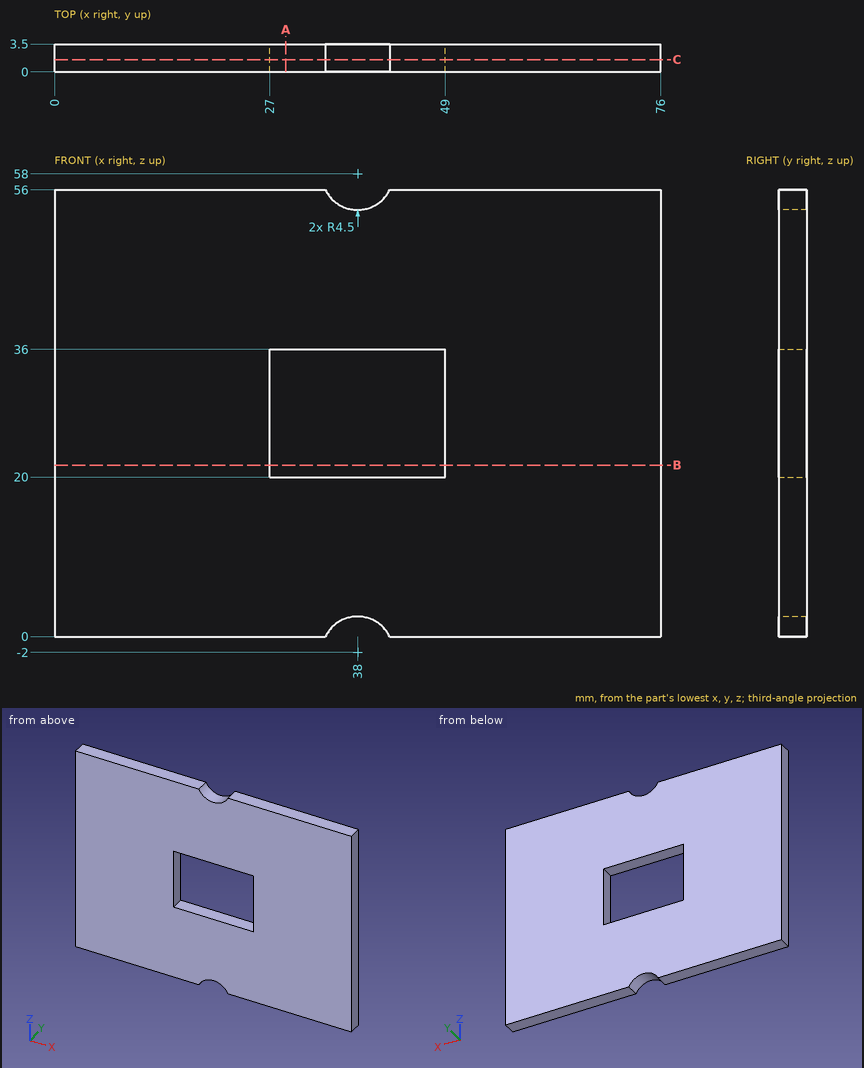
Here's the drawing with two shaded views (mm, measured from the low corner). I have some questions. Round coordinates to 2 decimals unless told otherwise and drop trailing zeros. Loops run counter-clockwise (first coordinate to the right, second up) from the corner with the lowest first, then second, coordinate; pieces in that order, holes last.
Item 1: Suppose I cut it at A-A, the plane x = 29. Write out the boundary of the cut face in (y, z).
Item 2: Suppose I cut it at C-C, the plane y = 1.55. Write out the boundary of the cut face in (x, z), then the cut area to 3 significant figures.
Item 3: Will these pins go through, and if not, where does the flat tip stop? pin 1 Ø1 at (x, y) = (38.5, 2.5) entering from +Z; pin 2 Ø1.8 at (x, y) = (39.5, 2.5) entering from -Z.
Item 4: Please list where these lines run through material, in increasing order: L1, parallel to X at y = 3.15, z = 35; L2, parallel to Z at x = 38, y = 1.15; L3, parallel to Z at x = 32, y = 1.5.
Item 5: Suppose I cut it at B-B, the plane z = 21.5. Write out the boundary of the cut face in (x, y), then the cut area to 3 significant figures.
Reported:
1. outline: (0, 0) - (3.5, 0) - (3.5, 20) - (0, 20) - close; (0, 36) - (3.5, 36) - (3.5, 56) - (0, 56) - close
2. outline: (0, 0) - (33.97, 0) arc R4.5 cw to (42.03, 0) - (76, 0) - (76, 56) - (42.03, 56) arc R4.5 cw to (33.97, 56) - (0, 56) - close; hole (27, 20) - (49, 20) - (49, 36) - (27, 36) - close
2. area: 3,880 mm2
3. pin 1: stops at z = 53.61
3. pin 2: stops at z = 1.81
4. L1: x = 0 to 27, 49 to 76
4. L2: z = 2.5 to 20, 36 to 53.5
4. L3: z = 0 to 20, 36 to 56
5. outline: (0, 0) - (27, 0) - (27, 3.5) - (0, 3.5) - close; (49, 0) - (76, 0) - (76, 3.5) - (49, 3.5) - close
5. area: 189 mm2
